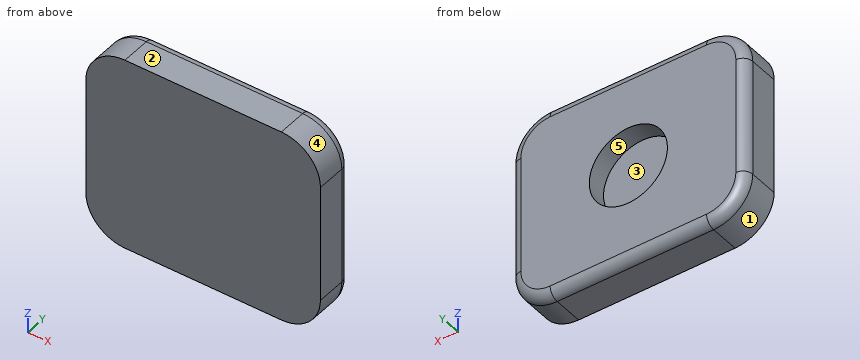
from build123d import *

# Parameters (mm, degrees)
SKETCH2_W           = 120
SKETCH2_H           = 100
SKETCH2_R           = 20
BOSS_EXTRUDE1_DEPTH = 10
SKETCH3_W           = 120
SKETCH3_H           = 100
BOSS_EXTRUDE2_DEPTH = 10
FILLET1_R           = 20
FILLET2_R           = 5


with BuildPart() as part:
    # Sketch2 → Boss-Extrude1 (new body)
    with BuildSketch(Plane(origin=(0, 0, 0), x_dir=(1, 0, 0), z_dir=(0, 1, 0))):
        Rectangle(SKETCH2_W, SKETCH2_H)
        with Locations(Location((0, 0, 0), (0, 0, 270))):
            Circle(SKETCH2_R, mode=Mode.SUBTRACT)
    extrude(amount=BOSS_EXTRUDE1_DEPTH)

    # Sketch3 → Boss-Extrude2 (add)
    with BuildSketch(Plane.XZ):
        Rectangle(SKETCH3_W, SKETCH3_H)
    extrude(amount=BOSS_EXTRUDE2_DEPTH)

    # Fillet1
    fillet1_edges = [part.edges().sort_by_distance(p)[0] for p in [
        (60, 0, 50),
        (-60, 0, 50),
        (-60, 0, -50),
        (60, 0, -50),
    ]]
    fillet(fillet1_edges, radius=FILLET1_R)

    # Fillet2
    fillet2_edges = [part.edges().sort_by_distance(p)[0] for p in [
        (-60, 10, 0),
        (0, 10, -50),
        (60, 10, 0),
        (0, 10, 50),
        (54.142135624, 10, 44.142135624),
        (54.142135624, 10, -44.142135624),
        (-54.142135624, 10, 44.142135624),
        (-54.142135624, 10, -44.142135624),
    ]]
    fillet(fillet2_edges, radius=FILLET2_R)


solid = part.part
Geometry: final body of the model. Coordinates: model frame, mm. Face numbers are marked on the shaded views. A direction names the side the tool comes from. Coordinates: 2 decimals unless noted, no trailing zeros. Loops run counter-clockwise (first coordinate to the right, second up) from the corner with the lowest first, then second, coordinate; pieces in that order, holes last. Notation, with made-up numbers: (16, 42.5) - (26, 42.5) arc R21 ccw to (26, 68.5) - close; hole circle Ø3 at (22.25, 78.5). An arc over 180 degrees is marked (long way). Put each result on its own line as item: value. Start each with the question number.
Q1. Cut plane B-B, the plane z = 0. Return loops of the section in (x, y), and give its area (3 significant figures).
Q2. Set-up query: the marked faces 4 and 5. Return all of +Z, -Z, +X, -X, +Y, -Y with unobstructed straight access to the full face (end or side cutting, diameter ignored); none if empty.
Q3. Cut plane A-A, the plane x = 0. Return loops of the section in (y, z), and give its area (3 significant figures).
Q4. Line query: line 1 (X direction, y = 3, z = 0); line 2 (X direction, y = 0.5, z = 18); line 3 (Z direction, x = -2.5, y = 8). Output: solid intervals per line, ascending.
Q5. Pin query (flat end, axial travel): pin 1 Ø10 at (y, z) = (3, 33) entering from +X; pin 2 Ø1.5 at (y, z) = (2, 38) entering from -X; pin 3 Ø20 at (x, z) = (1, 1) entering from +Y; pin 4 Ø2 at (x, y) = (-42.5, -6.5) entering from +Z. Return the tip coordinate at first contact, or that it passes through.
Q6. Pull-direction query (X, two-part tool) for the marked faces 1, 2 and 3; classes: released by +X, released by -X, zero draft, split by the parting line, or undercut.
Filled sheet:
1. outline: (-60, -10) - (60, -10) - (60, 5) arc R5 ccw to (55, 10) - (20, 10) - (20, 0) - (-20, 0) - (-20, 10) - (-55, 10) arc R5 ccw to (-60, 5) - close
1. area: 1,990 mm²
2. face 4: +Z, +X, +Y, -Y
2. face 5: +Y
3. outline: (-10, -50) - (5, -50) arc R5 ccw to (10, -45) - (10, -20) - (0, -20) - (0, 20) - (10, 20) - (10, 45) arc R5 ccw to (5, 50) - (-10, 50) - close
3. area: 1,590 mm²
4. line 1: -60 to -20, 20 to 60
4. line 2: -60 to -8.72, 8.72 to 60
4. line 3: -49 to -19.84, 19.84 to 49
5. pin 1: x = 60
5. pin 2: x = -58.64
5. pin 3: y = 0
5. pin 4: z = 49.94
6. face 1: released by -X
6. face 2: zero draft
6. face 3: undercut
